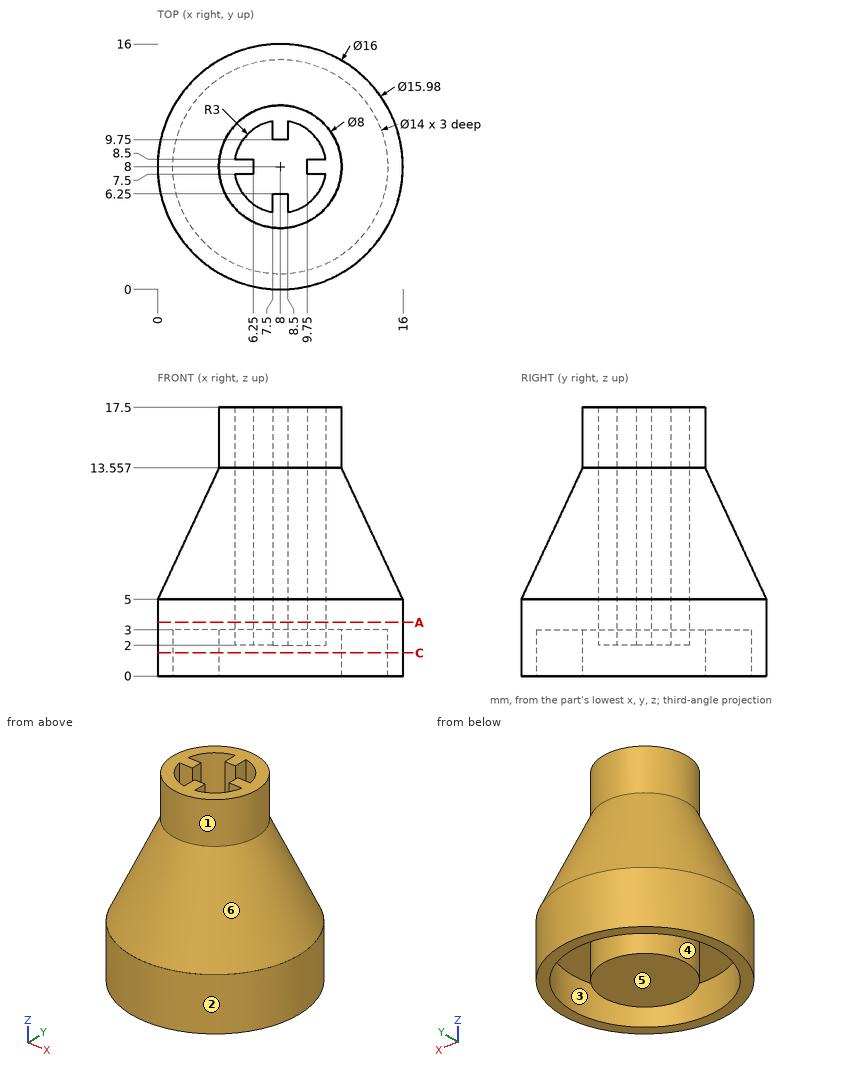
Can you work these out from the drawing? Everything is in mm from the part's minimum corner. A direction names the side the tool comes from. Coordinates: 2 decimals unless noted, no trailing zeros. Write each loop counter-clockwise with the first axis right and the second up, starting at its lowest first coordinate (ties: lowest second). Pieces come first, ordered by that corner, then holes. Notation, with made-up numbers: (20, 74) -> (45, 74) arc R23 ccw to (45, 102) -> close; hole circle Ø1 at (25, -37). An arc over 180 degrees is marked (long way). Write each question's results on one line, items separated by ' | '. Start each with the question number.
Q1. Imagine slicing it at A-A (z = 3.5). Write out the boundary of the cut face in (x, y).
Q2. If I drill on probe 1 along Y at (x, z) = (8, 1.3); probe 2 along Y at (x, z) = (8, 2.3); probe 3 along Y at (x, z) = (10, 11.25) (1 decimal), over which ranges is the centre line in solid material (lowest first)?
Q3. We'd pull the mould along Y, two halves only. Please class the marked faces 4, 5 and 6: +Y half, -Y half, draft (parallel to the pull), parting line (faces both ways), or undercut.
Q4. On a 3-axis mill with a long thin cutter (end or side, diameter ignored), from which of +Z, -Z, +X, -X, +Y, -Y can I reach the whole of each face in a straight line? I mean the marked faces 1, 2 and 3. Say none if no direction works.
Q5. Imagine slicing it at C-C (z = 1.5). Write out the boundary of the cut face in (x, y).
Q6. I'm going to push flat-ended pins straight in: pin 1 (1.1 mm diameter, centred on x = 8, z = 10.5, fed in from +Y); pin 2 (8 mm diameter, centred on y = 9, z = 4.5, fed in from -X); pin 3 (0.8 mm diameter, centred on x = 8, z = 10, fed in from -Y) (1 decimal); pin 4 (1 mm diameter, centred on x = 13.5, y = 8.5, fed in from -Z). Where does each tip first touch, or does it pass through?
Taken from the geometry:
1) outline: circle Ø16 at (8, 8); hole (5.04, 7.5) arc R3 ccw to (7.5, 5.04) -> (7.5, 6.25) -> (8.5, 6.25) -> (8.5, 5.04) arc R3 ccw to (10.96, 7.5) -> (9.75, 7.5) -> (9.75, 8.5) -> (10.96, 8.5) arc R3 ccw to (8.5, 10.96) -> (8.5, 9.75) -> (7.5, 9.75) -> (7.5, 10.96) arc R3 ccw to (5.04, 8.5) -> (6.25, 8.5) -> (6.25, 7.5) -> close
2) probe 1: y = 0 to 1, 4 to 12, 15 to 16 | probe 2: y = 0 to 1, 4 to 6.25, 9.75 to 12, 15 to 16 | probe 3: y = 3.3 to 5.8, 7.5 to 8.5, 10.2 to 12.7
3) face 4: undercut | face 5: draft | face 6: parting line
4) face 1: +Z | face 2: +Z, -Z | face 3: -Z
5) outline: circle Ø16 at (8, 8); circle Ø8 at (8, 8); hole circle Ø14 at (8, 8)
6) pin 1: stops at y = 13.68 | pin 2: stops at x = 0 | pin 3: stops at y = 2.2 | pin 4: stops at z = 3
